Autodesk Inventor part; units mm, degrees
ref_plane "YZ Plane" through (0, 0, 0) normal (1, 0, 0) x (0, 1, 0)
ref_plane "XZ Plane" through (0, 0, 0) normal (0, 1, 0) x (-1, 0, 0)
ref_plane "XY Plane" through (0, 0, 0) normal (0, 0, 1) x (1, 0, 0)
sketch "Sketch1" plane through (0, 0, 0) normal (0, 1, 0) x (-1, 0, 0)
  circle A0 centre (0, 0) radius 10
  circle A1 centre (0, 0) radius 12.5
  line L0 (12.5, 0) -> (12.5, 50)
  line L1 (-12.5, 0) -> (-12.5, 50)
  line L2 (-12.5, 50) -> (12.5, 50)
  dimension "d0" = 20
  dimension "d1" = 25
  dimension "d2" = 50
extrude "Extrusion1" add sketch "Sketch1" along normal blind 15
sketch "Sketch2" plane through (-12.5, 0, 0) normal (-1, 0, 0) x (0, 0, 1)
  line L0 (-12.5, 0) -> (-12.5, 15)
  line L1 (-12.5, 7.5) -> (37.5, 7.5)
  line L2 (25, 7.5) -> (25, 4.5)
  line L3 (25, 4.5) -> (25, 10.5)
  line L4 (25, 10.5) -> (75, 10.5)
  line L5 (75, 10.5) -> (75, 4.5)
  line L6 (75, 4.5) -> (25, 4.5)
  point P0 (0, 0)
  dimension "d5" = 50
  dimension "d8" = 3
  dimension "d9" = 6
  dimension "d10" = 50
extrude "Extrusion2" add sketch "Sketch2" along normal blind 10
sketch "Sketch3" plane through (-12.5, 0, 50) normal (0, 0, 1) x (1, 0, 0)
  point P0 (12.5, 0)
sketch "Sketch4" plane through (-12.5, 0, 50) normal (0, 0, 1) x (1, 0, 0)
  line L0 (25, 0) -> (25, 15)
  line L1 (25, 0) -> (25, 15)
  line L2 (0, 15) -> (25, 15)
  line L3 (25, 15) -> (0, 15)
  line L4 (0, 0) -> (0, 15)
  line L5 (0, 15) -> (0, 0)
  line L6 (0, 0) -> (25, 0)
  line L7 (0, 0) -> (25, 0)
  point P0 (12.5, 0)
extrude "Extrusion3" add sketch "Sketch4" along normal blind 25
sketch "Sketch5" plane through (-12.5, 4.5, 25) normal (0, -1, 0) x (1, 0, 0)
  point P0 (12.5, -25)
sketch "Sketch6" plane through (-12.5, 4.5, 25) normal (0, -1, 0) x (1, 0, 0)
  line L0 (0, 0) -> (-10, 0)
  line L1 (-5, 0) -> (-5, 50)
  line L2 (0, 50) -> (-10, 50)
  line L3 (-5, 0) -> (-5, 10)
  line L4 (-3.75, 8.75) -> (-6.25, 8.75)
  line L5 (-6.25, 8.75) -> (-6.25, 11.25)
  line L6 (-6.25, 11.25) -> (-3.75, 11.25)
  line L7 (-3.75, 11.25) -> (-3.75, 8.75)
  line L8 (-3.75, 8.75) -> (-6.25, 11.25) construction
  line L9 (-6.25, 8.75) -> (-3.75, 11.25) construction
  line L10 (-5, 11.25) -> (-5, 15.25)
  line L11 (-3.75, 15.25) -> (-6.25, 15.25)
  line L12 (-6.25, 15.25) -> (-6.25, 17.75)
  line L13 (-6.25, 17.75) -> (-3.75, 17.75)
  line L14 (-3.75, 17.75) -> (-3.75, 15.25)
  point P0 (12.5, -25)
  dimension "d15" = 10
  dimension "d16" = 2.5
  dimension "d17" = 2.5
  dimension "d18" = 4
  dimension "d19" = 2.5
sketch "Sketch7" plane through (-12.5, 4.5, 25) normal (0, -1, 0) x (1, 0, 0)
  line L0 (-4.9925, 17.7874) -> (-4.9925, 21.7874)
  line L1 (-4.9925, 21.7874) -> (-3.7425, 21.7874)
  line L2 (-3.7425, 21.7874) -> (-3.7425, 24.2874)
  line L3 (-3.7425, 24.2874) -> (-6.2425, 24.2874)
  line L4 (-6.2425, 24.2874) -> (-6.2425, 21.7874)
  line L5 (-6.2425, 21.7874) -> (-4.9925, 21.7874)
  line L6 (-4.9925, 24.2874) -> (-4.9925, 28.2874)
  line L7 (-4.9925, 28.2874) -> (-6.2425, 28.2874)
  line L8 (-6.2425, 28.2874) -> (-6.2425, 30.7874)
  line L9 (-6.2425, 30.7874) -> (-3.7425, 30.7874)
  line L10 (-3.7425, 30.7874) -> (-3.7425, 28.2874)
  line L11 (-4.9925, 28.2874) -> (-3.7425, 28.2874)
  line L12 (-4.9925, 30.7874) -> (-4.9925, 34.7874)
  line L13 (-4.9925, 34.7874) -> (-3.7425, 34.7874)
  line L14 (-3.7425, 34.7874) -> (-3.7425, 37.2874)
  line L15 (-3.7425, 37.2874) -> (-6.2425, 37.2874)
  line L16 (-6.2425, 37.2874) -> (-6.2425, 34.7874)
  line L17 (-6.2425, 34.7874) -> (-4.9925, 34.7874)
  line L18 (-4.9925, 37.2874) -> (-4.9925, 41.2874)
  line L19 (-4.9925, 41.2874) -> (-3.7425, 41.2874)
  line L20 (-3.7425, 41.2874) -> (-3.7425, 43.7874)
  line L21 (-3.7425, 43.7874) -> (-6.2425, 43.7874)
  line L22 (-6.2425, 43.7874) -> (-6.2425, 41.2874)
  line L23 (-6.2425, 41.2874) -> (-4.9925, 41.2874)
  line L24 (-5, 15.2622) -> (-5, 8.7622)
  line L25 (-5, 8.7622) -> (-5, 4.7622)
  line L26 (-5, 4.7622) -> (-6.25, 4.7622)
  line L27 (-6.25, 4.7622) -> (-6.25, 2.2622)
  line L28 (-6.25, 2.2622) -> (-3.75, 2.2622)
  line L29 (-3.75, 2.2622) -> (-3.75, 4.7622)
  line L30 (-3.75, 4.7622) -> (-5, 4.7622)
  point P0 (12.5, -25)
  dimension "d20" = 4
  dimension "d21" = 1.25
  dimension "d22" = 2.5
  dimension "d23" = 2.5
  dimension "d24" = 4
  dimension "d25" = 1.25
  dimension "d26" = 2.5
  dimension "d27" = 4
  dimension "d28" = 2.5
  dimension "d29" = 4
  dimension "d30" = 2.5
  dimension "d31" = 6.5
  dimension "d32" = 4
  dimension "d33" = 1.25
  dimension "d34" = 2.5
  dimension "d35" = 2.5
Model file for the job. Use its own axes, mm. A direction names the side the tool comes from. Coordinates: 2 decimals unless noted, no trailing zeros. Order: outer loops, then holes, each group sorted by start corner. A loop starts at its lowest first (then second) coordinate and runs counter-clockwise, first axis right, second up. Notation, with made-up numbers: (88.5, 52.25) - (142.5, 52.25) arc R17 ccw to (142.5, 61.25) - close; hole circle Ø7 at (76, 74). An arc over 180 degrees is marked (long way). Return JSON: item names as keys, results as strings. Group by question number.
1) Saw through at B-B, the plane z = 30.5. Write the cut outline in (x, y), plus the area to 3 significant figures.
2) Saw through at C-C, the plane y = 2. Write the cut outline in (x, z), plus the area to 3 significant figures.
3) Flat gauge pins, fed straight in: P1, Ø1.8, axis at x = -17, y = 6.5, coming from the -Z side; P2, Ø5, axis at x = -18.5, z = 41.5, coming from the +Y side; P3, Ø1.5, axis at y = 12, z = 57.5, coming from the -X side. Where does each tip first touch, or does it go through?
4) Saw through at D-D, the plane z = -4.5. Write the cut outline in (x, y).
5) Mould opens along Z. For faces 5 (the cylindrical face through (2.17, 7.4, 9.76)), 6 (the flat face through (-12.5, 4, 37)), 7 (the flat face through (-1, 8, 75)) say: released by +Z, released by -Z, zero draft, split by the parting line, or undercut.
6) Tool access for faces 1 (the flat face through (-17, 10.5, 50)), 2 (the flat face through (-17, 4.5, 50)), 3 (the flat face through (-17, 7, 25)), 4 (the cylindrical face through (-0.275, 7.395, -12.497)): list every direction of +Z, -Z, +X, -X, +Y, -Y with a clear straight run to the whole face (end or side of a thin tool).
7) Probe line 1 (Z direction, x = 0, y = 9.75); line 2 (X direction, y = 2, z = 0.5); line 3 (X direction, y = 6.75, z = 8). List the from-to ranges inside material, lowest first. Write a range as from..to.
8) Saw through at A-A, the plane x = 0. Write the cut outline in (y, z), plus the area to 3 significant figures.
Values found:
{
 "1": {"outline": "(-22.5, 4.5) - (-12.5, 4.5) - (-12.5, 0) - (12.5, 0) - (12.5, 15) - (-12.5, 15) - (-12.5, 10.5) - (-22.5, 10.5) - close", "area": "435 mm²"},
 "2": {"outline": "(-12.5, 0) arc R12.5 ccw to (12.5, 0) - (12.5, 75) - (-12.5, 75) - close; hole circle Ø20 at (0, 0)", "area": "1,810 mm²"},
 "3": {"P1": "stops at z = 25", "P2": "stops at y = 10.5", "P3": "stops at x = -12.5"},
 "4": {"outline": "(-11.66, 0) - (-8.93, 0) - (-8.93, 15) - (-11.66, 15) - close; (8.93, 0) - (11.66, 0) - (11.66, 15) - (8.93, 15) - close"},
 "5": {"face 5": "undercut", "face 6": "zero draft", "face 7": "released by +Z"},
 "6": {"face 1": "+Z, -Z, -X, +Y", "face 2": "+Z, -Z, -X, -Y", "face 3": "-Z, -X, +Y, -Y", "face 4": "-Z, +Y, -Y"},
 "7": {"line 1": "z = -12.5..-10, 10..75", "line 2": "x = -12.5..-9.99, 9.99..12.5", "line 3": "x = -12.5..-6, 6..12.5"},
 "8": {"outline": "(0, -12.5) - (15, -12.5) - (15, -10) - (0, -10) - close; (0, 10) - (15, 10) - (15, 75) - (0, 75) - close", "area": "1,010 mm²"}
}
